from build123d import *

# Parameters (mm, degrees)
SKETCH1_W                       = 30.734
SKETCH1_H                       = 196.596
BOSS_EXTRUDE1_DEPTH             = 0.0254
SKETCH22_W                      = 30.734
SKETCH22_H                      = 196.596
BOSS_EXTRUDE10_DEPTH            = 5.08
BOSS_EXTRUDE11_DEPTH            = 127
FILLET1_R                       = 7.62
BOSS_EXTRUDE3_REACH             = 227.812
SKETCH6_W                       = 6.35
SKETCH6_H                       = 132.08
BOSS_EXTRUDE3_DIRECTION_2_REACH = 227.812
BOSS_EXTRUDE7_REACH             = 238.982
SKETCH19_W                      = 19.05
SKETCH19_H                      = 19.05
CUT_EXTRUDE2_DEPTH              = 240.465115736
SKETCH20_W                      = 135.918968774
SKETCH20_H                      = 500.058977118
CUT_EXTRUDE3_DEPTH              = 153.162
CUT_EXTRUDE5_DEPTH              = 240.512169756
CUT_EXTRUDE6_DEPTH              = 248.87835803
CUT_EXTRUDE6_DEPTH_BACK         = 248.87835803
SKETCH29_W                      = 0.508
SKETCH29_H                      = 309.433656838
SKETCH29_H_2                    = 1270


with BuildPart() as part:
    # Sketch1 → Boss-Extrude1 (new body)
    with BuildSketch(Plane(origin=(0, 0, 0), x_dir=(1, 0, 0), z_dir=(0, 1, 0))):
        with Locations((15.367, 98.298)):
            Rectangle(SKETCH1_W, SKETCH1_H)
    extrude(amount=BOSS_EXTRUDE1_DEPTH)

    # Sketch22 → Boss-Extrude10 (add)
    with BuildSketch(Plane.XZ):
        with Locations((15.367, -98.298)):
            Rectangle(SKETCH22_W, SKETCH22_H)
    extrude(amount=BOSS_EXTRUDE10_DEPTH)

    # Sketch23 → Boss-Extrude11 (add)
    with BuildSketch(Plane(origin=(0, 0.0254, 0), x_dir=(1, 0, 0), z_dir=(0, 1, 0))):
        Polygon((0, 183.896), (6.35, 183.896), (12.7, 190.246), (18.034, 190.246), (24.384, 183.896), (30.734, 183.896), (30.734, 196.596), (0, 196.596), align=None)
        Polygon((30.734, 0), (6.350000064, 0), (6.366832231, 12.699988846), (12.716832231, 12.699988846), (16.383, 6.35), (18.923, 6.35), (24.384, 12.7), (30.734, 12.7), align=None)
    extrude(amount=BOSS_EXTRUDE11_DEPTH)

    # Fillet1
    # the kernel refuses this fillet: 7.62 mm, written as the material it takes off along each edge
    with BuildSketch(Plane(origin=(6.366832231, 0.0254, -12.699988846), x_dir=(1, 0, 0), z_dir=(0, 1, 0))) as fillet1_piece_1:
        with BuildLine():
            CenterArc((7.610046419, -7.515097007), FILLET1_R, 99.518172774, 80.405889243)
            Line((-0.009946888, -7.504997707), (0, 0))
            Line((0, 0), (6.35, 0))
        make_face()
    extrude(amount=145.762510746, mode=Mode.SUBTRACT)

    # Boss-Extrude3: up to this face of the body (flat: up to its plane)
    boss_extrude3_end = Plane(part.part.faces().sort_by_distance((18.388884901, 60.339992847, 0))[0])
    # Sketch6 → Boss-Extrude3 (add, up to the picked face)
    with BuildSketch(Plane.XY.offset(-184.15), mode=Mode.PRIVATE) as boss_extrude3_sk1:
        with Locations((33.909, 60.9854)):
            Rectangle(SKETCH6_W, SKETCH6_H)
    boss_extrude3_tool1 = split(extrude(boss_extrude3_sk1.sketch, amount=BOSS_EXTRUDE3_REACH, mode=Mode.PRIVATE), bisect_by=boss_extrude3_end, keep=Keep.BOTH, mode=Mode.PRIVATE)
    add(boss_extrude3_tool1.solids().sort_by(Axis((33.909, 60.9854, -184.15), (0, 0, 1)))[0])

    # Boss-Extrude3 direction 2: up to this face of the body (flat: up to its plane)
    boss_extrude3_direction_2_end = Plane(part.part.faces().sort_by_distance((15.367, 60.9727, -196.596))[0])
    # Sketch6 → Boss-Extrude3 direction 2 (add, up to the picked face)
    with BuildSketch(Plane.XY.offset(-184.15), mode=Mode.PRIVATE) as boss_extrude3_direction_2_sk1:
        with Locations((33.909, 60.9854)):
            Rectangle(SKETCH6_W, SKETCH6_H)
    boss_extrude3_direction_2_tool1 = split(extrude(boss_extrude3_direction_2_sk1.sketch, amount=-BOSS_EXTRUDE3_DIRECTION_2_REACH, mode=Mode.PRIVATE), bisect_by=boss_extrude3_direction_2_end, keep=Keep.BOTH, mode=Mode.PRIVATE)
    add(boss_extrude3_direction_2_tool1.solids().sort_by(Axis((33.909, 60.9854, -184.15), (0, 0, -1)))[0])

    # Boss-Extrude7: up to this face of the body (flat: up to its plane)
    boss_extrude7_end = Plane(part.part.faces().sort_by_distance((18.541494055, 60.974874311, -196.596))[0])
    # Sketch15 → Boss-Extrude7 (add, up to the picked face)
    with BuildSketch(Plane.XY, mode=Mode.PRIVATE) as boss_extrude7_sk1:
        Polygon((-50.8, -8.87193717), (-49.680323673, -15.22193717), (39.219676327, 0.453531415), (38.1, 6.803531415), align=None)
    boss_extrude7_tool1 = split(extrude(boss_extrude7_sk1.sketch, amount=-BOSS_EXTRUDE7_REACH, mode=Mode.PRIVATE), bisect_by=boss_extrude7_end, keep=Keep.BOTH, mode=Mode.PRIVATE)
    add(boss_extrude7_tool1.solids().sort_by(Axis((-5.790162, -4.209203, 0), (0, 0, -1)))[0])

    # Sketch19 → Cut-Extrude2 (cut, through all)
    with BuildSketch(Plane(origin=(-0.014616821, 0.08289611, 0), x_dir=(0.984807753012208, 0.1736481776669311, 0), z_dir=(-0.1736481776669311, 0.984807753012208, 0))):
        with Locations((-22.993829575, 168.021)):
            Rectangle(SKETCH19_W, SKETCH19_H)
        with Locations((-22.993829575, 142.621)):
            Rectangle(SKETCH19_W, SKETCH19_H)
        with Locations((-22.993829575, 117.221)):
            Rectangle(SKETCH19_W, SKETCH19_H)
        with Locations((-22.993829575, 91.821)):
            Rectangle(SKETCH19_W, SKETCH19_H)
        with Locations((-22.993829575, 66.421)):
            Rectangle(SKETCH19_W, SKETCH19_H)
    extrude(amount=-CUT_EXTRUDE2_DEPTH, mode=Mode.SUBTRACT)

    # Sketch20 → Cut-Extrude3 (cut)
    with BuildSketch(Plane(origin=(1.105059507, -6.26710389, 0), x_dir=(0.9848077530122079, 0.17364817766693127, 0), z_dir=(0.17364817766693127, -0.9848077530122079, 0))):
        with Locations((20.082569743, -64.610703306)):
            Rectangle(SKETCH20_W, SKETCH20_H)
    extrude(amount=CUT_EXTRUDE3_DEPTH, mode=Mode.SUBTRACT)

    # Sketch28 → Cut-Extrude5 (cut, through all)
    with BuildSketch(Plane.XY):
        Polygon((39.219676327, 0.453531415), (38.1, 6.803531415), (37.084, 6.624383203), (37.848330327, 0.211726115), align=None)
    extrude(amount=-CUT_EXTRUDE5_DEPTH, mode=Mode.SUBTRACT)

    # Sketch29 → Cut-Extrude6 (cut, two sides: drawn at the far end of the back side and taken through both)
    with BuildSketch(Plane(origin=(37.343053222, 4.450951877, 0), x_dir=(0, 0, -1), z_dir=(0.992971564369303, 0.11835316790850746, 0)).offset(-CUT_EXTRUDE6_DEPTH_BACK)):
        with Locations((0.254, 29.905643692)):
            Rectangle(SKETCH29_W, SKETCH29_H)
        with Locations((196.342, 626.49740635)):
            Rectangle(SKETCH29_W, SKETCH29_H_2)
    extrude(amount=CUT_EXTRUDE6_DEPTH + CUT_EXTRUDE6_DEPTH_BACK, mode=Mode.SUBTRACT)


solid = part.part
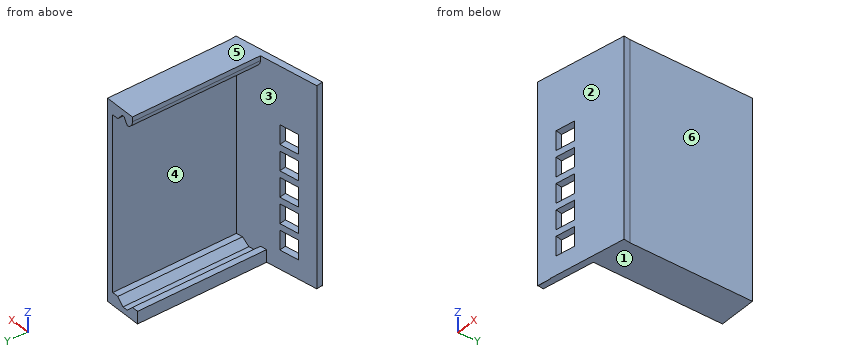
Input: part model. Units: mm. Frame: model coordinates. Face numbers are marked on the shaded views. A direction names the side the tool comes from. Give positions to 0.01 mm unless a question says otherwise; leave off trailing zeros. Order: outer loops, then holes, each group sorted by start corner. A loop starts at its lowest first (then second) coordinate and runs counter-clockwise, first axis right, second up.
Q1. Section A-A on z = -123. Output: boundary loops of the cut face in (x, y).
Checked values:
outline: (-50.8, -8.87) - (-49.68, -15.22) - (-30.92, -11.91) - (-32.04, -5.56) - close; (-13.28, -2.26) - (-12.16, -8.61) - (37.85, 0.21) - (37.08, 6.62) - (37.08, 127.03) - (30.73, 127.03) - (30.73, 5.5) - close
Q2. Contact query for flat-ended pins moving along their axis: pin 1 Ø1.5 at (x, z) = (-31.5, -105) entering from +Y; pin 2 Ø5 at (x, y) = (-26, -6) entering from -Z; pin 3 Ø3 at (x, z) = (6, -26.5) entering from -Y. Output: stop coordinate, or through.
Checked values:
pin 1: stops at y = -5.34
pin 2: stops at z = -196.09
pin 3: stops at y = -5.67
Q3. Section B-B on x = -22. Output: boundary loops of the cut face in (y, z), and give its area (3 significant figures).
Checked values:
outline: (-10.34, -196.09) - (-3.79, -196.09) - (-3.79, -177.55) - (-10.34, -177.55) - close; (-10.34, -158.5) - (-3.79, -158.5) - (-3.79, -152.15) - (-10.34, -152.15) - close; (-10.34, -133.1) - (-3.79, -133.1) - (-3.79, -126.75) - (-10.34, -126.75) - close; (-10.34, -107.7) - (-3.79, -107.7) - (-3.79, -101.35) - (-10.34, -101.35) - close; (-10.34, -82.3) - (-3.79, -82.3) - (-3.79, -75.95) - (-10.34, -75.95) - close; (-10.34, -56.9) - (-3.79, -56.9) - (-3.79, -0.51) - (-10.34, -0.51) - close
area: 657 mm2
Q4. Section D-D on z = -36. Output: boundary loops of the cut face in (x, y).
Checked values:
outline: (-50.8, -8.87) - (-49.68, -15.22) - (37.85, 0.21) - (37.08, 6.62) - (37.08, 127.03) - (30.73, 127.03) - (30.73, 5.5) - close
Q5. Ray query, probe 1 along Z at (x, y) = (26, 60); probe 2 along X at (y, z) = (53, -165); probe 3 along Z at (x, y) = (1, 100.5). Return the intervals inside material, ascending.
Checked values:
probe 1: z = -196.09 to -183.9, -12.7 to -0.51
probe 2: x = 30.73 to 37.08
probe 3: z = -196.09 to -183.9
Q6. Section C-C on y = 109. Output: boundary loops of the cut face in (x, z) (3 decimals), and give its area (3 significant figures).
Checked values:
outline: (0, -196.088) - (37.084, -196.088) - (37.084, -0.508) - (6.351, -0.508) - (6.357, -5.195) arc R7.62 ccw to (12.717, -12.7) - (16.383, -6.35) - (18.923, -6.35) - (24.384, -12.7) - (30.734, -12.7) - (30.734, -183.896) - (24.384, -183.896) - (18.034, -190.246) - (12.7, -190.246) - (6.35, -183.896) - (0, -183.896) - close
area: 1,780 mm2
Q7. Draft query along Z for the marked faces 1, 2 and 3. Return one class per face: +Z half, -Z half, draft (parallel to the pull), parting line (faces both ways), or undercut.
Checked values:
face 1: -Z half
face 2: draft
face 3: undercut
Q8. Set-up query: the marked faces 4, 5 and 6. Return all of +Z, -Z, +X, -X, +Y, -Y with unobstructed straight access to the full face (end or side cutting, diameter ignored); none if empty.
Checked values:
face 4: -X, +Y
face 5: +Z, +X, -X, +Y, -Y
face 6: +Z, -Z, +X, +Y
